from build123d import *

# Parameters (mm, degrees)
F0_W     = 12
F0_H     = 12
F1_DEPTH = 4.83
F3_DEPTH = 25
F4_R     = 1


with BuildPart() as f1:
    # F0 (on Top) → F1 (new body)
    with BuildSketch(Plane.XY):
        Rectangle(F0_W, F0_H)
    extrude(amount=F1_DEPTH)

    # F2 (on face) → F3 (cut)
    with BuildSketch(Plane.XZ.offset(6)):
        Polygon((4.5, 2.323068), (4.5, 1), (6, 1), (6, 4.83), (0, 4.83), (0, 4.323068), (1.5, 4.323068), (1.5, 3.323068), (3, 3.323068), (3, 2.323068), align=None)
    extrude(amount=-F3_DEPTH, mode=Mode.SUBTRACT)

    # F4
    f4_edges = [f1.edges().sort_by_distance(p)[0] for p in [
        (-6, -6, 2.415),
        (-6, 6, 2.415),
        (6, -6, 0.5),
        (6, 6, 0.5),
    ]]
    fillet(f4_edges, radius=F4_R)


solid = f1.part
Model file for the job. Use its own axes, mm. A direction names the side the tool comes from. Give positions to 0.01 mm unless a question says otherwise; leave off trailing zeros. Write each loop counter-clockwise with the first axis right and the second up, starting at its lowest first coordinate (ties: lowest second). Pieces come first, ordered by that corner, then holes. Notation, with made-up numbers: M 31,28.25 L 37,28.25 A24 ccw 37,40.25 Z; hole C -21.5,34 d2. An arc over 180 degrees is marked long. One line per item, written item: value. Start each with the question number.
Q1. Probe probe 1 along X at (y, z) = (0, 4.4); probe 2 along X at (y, z) = (4.5, 2.6); probe 3 along Z at (x, y) = (0.5, -0.25). List the from-to ranges inside material, lowest first. Write a range as [from, to].
Q2. Saw through at C-C, the plane x = 2.75. Write the cut outline in (y, z), plus the area to 3 significant figures.
Q3. Saw through at D-D, the plane z = 2.8. Write the cut outline in (x, y), plus the area to 3 significant figures.
Q4. Saw through at A-A, the plane z = 2.1. Write the cut outline in (x, y).
Q5. 3-axis set-ups, long thin cutter, end or side, ignore diameter. For faces 1 (the flat face through (5, 0, 1)), 2 (the flat face through (-1, 6, 2)): which of +Z, -Z, +X, -X, +Y, -Y reach the whole face in a straight line?
Q6. Drop flat-ended pins along their axis: pin 1 Ø0.8 at (x, y) = (2, -0.5) entering from +Z; pin 2 Ø0.5 at (y, z) = (-2.5, 3.5) entering from +X; pin 3 Ø0.8 at (x, y) = (5.5, 1) entering from +Z. Give the stop position or say it passes through.
Q7. Saw through at B-B, the plane y = 1. Write the cut outline in (x, z).
Output values:
1. probe 1: x = [-6, 0]
1. probe 2: x = [-6, 3]
1. probe 3: z = [0, 4.32]
2. outline: M -6,0 L 6,0 L 6,3.32 L -6,3.32 Z
2. area: 39.9 mm²
3. outline: M -6,-5 A1 ccw -5,-6 L 3,-6 L 3,6 L -5,6 A1 ccw -6,5 Z
3. area: 108 mm²
4. outline: M -6,-5 A1 ccw -5,-6 L 4.5,-6 L 4.5,6 L -5,6 A1 ccw -6,5 Z
5. face 1: +Z, +X, +Y, -Y
5. face 2: +Z, -Z, +X, -X, +Y
6. pin 1: stops at z = 3.32
6. pin 2: stops at x = 3
6. pin 3: stops at z = 1
7. outline: M -6,0 L 6,0 L 6,1 L 4.5,1 L 4.5,2.32 L 3,2.32 L 3,3.32 L 1.5,3.32 L 1.5,4.32 L 0,4.32 L 0,4.83 L -6,4.83 Z
